```python
from build123d import *

# Parameters (mm, degrees)
SKETCH2_R          = 1.25
ROTOR_HOLES_DEPTH  = 10
SKETCH4_R          = 1.75
STATOR_HOLES_DEPTH = 10
SKETCH5_R          = 1.75
HOLE_DEPTH         = 5
FILLET1_R          = 1
SKETCH6_R          = 1.5
SHAFT_DEPTH        = 7
CHAMFER1_SIZE      = 5


with BuildPart() as part:
    # Sketch1 → Body (revolve)
    with BuildSketch(Plane(origin=(0, 0, 0), x_dir=(0, 0, -1), z_dir=(1, 0, 0)), mode=Mode.PRIVATE) as body_sk:
        Polygon((0, 46), (-28, 46), (-39, 20), (-39, 0), (0, 0), align=None)
    revolve(body_sk.sketch.rotate(Axis((0, 0, 1764.481038956), (0, 0, -1)), 90), axis=Axis((0, 0, 1764.481038956), (0, 0, -1)))

    # Sketch2 → Rotor_Holes (cut)
    with BuildSketch(Plane.XY.offset(39)):
        with Locations((-11.25, 11.25)):
            Circle(SKETCH2_R)
        with Locations((11.25, 11.25)):
            Circle(SKETCH2_R)
        with Locations((11.25, -11.25)):
            Circle(SKETCH2_R)
        with Locations((-11.25, -11.25)):
            Circle(SKETCH2_R)
    extrude(amount=-ROTOR_HOLES_DEPTH, mode=Mode.SUBTRACT)

    # Sketch4 → Stator_Holes (cut)
    with BuildSketch(Plane(origin=(0, 0, 0), x_dir=(-1, 0, 0), z_dir=(0, 0, -1))):
        with Locations((-14.25, 14.25)):
            Circle(SKETCH4_R)
        with Locations((14.25, 14.25)):
            Circle(SKETCH4_R)
        with Locations((14.25, -14.25)):
            Circle(SKETCH4_R)
        with Locations((-14.25, -14.25)):
            Circle(SKETCH4_R)
    extrude(amount=-STATOR_HOLES_DEPTH, mode=Mode.SUBTRACT)

    # Sketch5 → Hole (cut)
    with BuildSketch(Plane(origin=(0, 0, 0), x_dir=(-1, 0, 0), z_dir=(0, 0, -1))):
        Circle(SKETCH5_R)
    extrude(amount=-HOLE_DEPTH, mode=Mode.SUBTRACT)

    # Fillet1
    fillet1_edges = [part.edges().sort_by_distance(p)[0] for p in [
        (1.75, 0, 0),
    ]]
    fillet(fillet1_edges, radius=FILLET1_R)

    # Sketch6 → Shaft (add)
    with BuildSketch(Plane.XY.offset(39)):
        with Locations(Location((0, 0, 0), (0, 0, 180))):
            Circle(SKETCH6_R)
    extrude(amount=SHAFT_DEPTH)

    # Chamfer1
    chamfer1_edges = [part.edges().sort_by_distance(p)[0] for p in [
        (-46, 0, 0),
    ]]
    chamfer(chamfer1_edges, length=CHAMFER1_SIZE)


solid = part.part
```
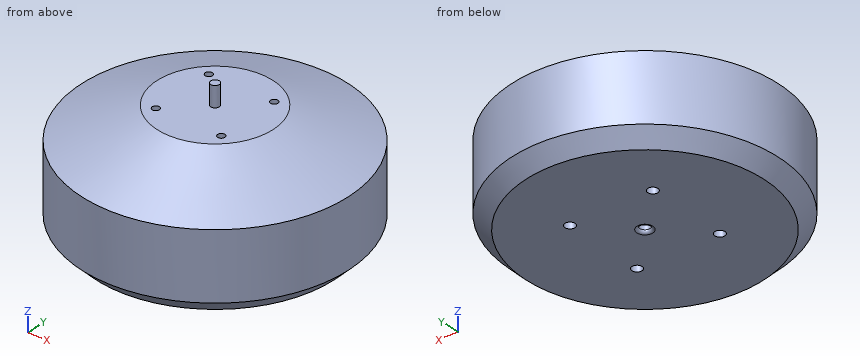
CAD build for the part. Positions are in the model's coordinates, mm. Coordinates: 2 decimals unless noted, no trailing zeros. Loops run counter-clockwise (first coordinate to the right, second up) from the corner with the lowest first, then second, coordinate; pieces in that order, holes last. Notation, with made-up numbers: (-31, 30.5) - (-3, 30.5) arc R19 cw to (-3, 45.5) - close; hole circle Ø3 at (-15.75, 29). An arc over 180 degrees is marked (long way). Use CSV: the item, a comma, the result in double quotes. Start each with the question number.
Q1. Probe probe 1 along Y at (x, z) = (-14, 5); probe 2 along X at (y, z) = (-11, 33); probe 3 along X at (y, z) = (11, 32). List the from-to ranges inside material, lowest first. Write a range as from..to.
Q2. Cut at C-C, the plane z = 43. List the corners of the cut face in (x, y).
Q3. Drop flat-ended pins along their axis: P1, Ø2, axis at y = -5.5, z = 36.5, coming from the -X side; P2, Ø12, axis at x = 9, y = -9, coming from the +Z side; P3, Ø3, axis at x = 0, y = 0, coming from the -Z side; P4, Ø4, axis at x = -0.5, y = -0.5, coming from the -Z side. Give the stop position or say it passes through.
Q4. Cut at A-A, the plane x = 0. List the corners of the cut face in (y, z).
Here are the results:
1,probe 1,"-43.82..-15.98, -12.52..12.52, 15.98..43.82"
1,probe 2,"-32.36..-12.47, -10.03..10.03, 12.47..32.36"
1,probe 3,"-34.85..-12.47, -10.03..10.03, 12.47..34.85"
2,outline,"circle Ø3 at (0, 0)"
3,P1,"x = -27.74"
3,P2,"z = 39"
3,P3,"z = 5"
3,P4,"z = 0"
4,outline,"(-46, 5) - (-41, 0) - (-2.75, 0) arc R1 ccw to (-1.75, 1) - (-1.75, 5) - (1.75, 5) - (1.75, 1) arc R1 ccw to (2.75, 0) - (41, 0) - (46, 5) - (46, 28) - (20, 39) - (1.5, 39) - (1.5, 46) - (-1.5, 46) - (-1.5, 39) - (-20, 39) - (-46, 28) - close"
